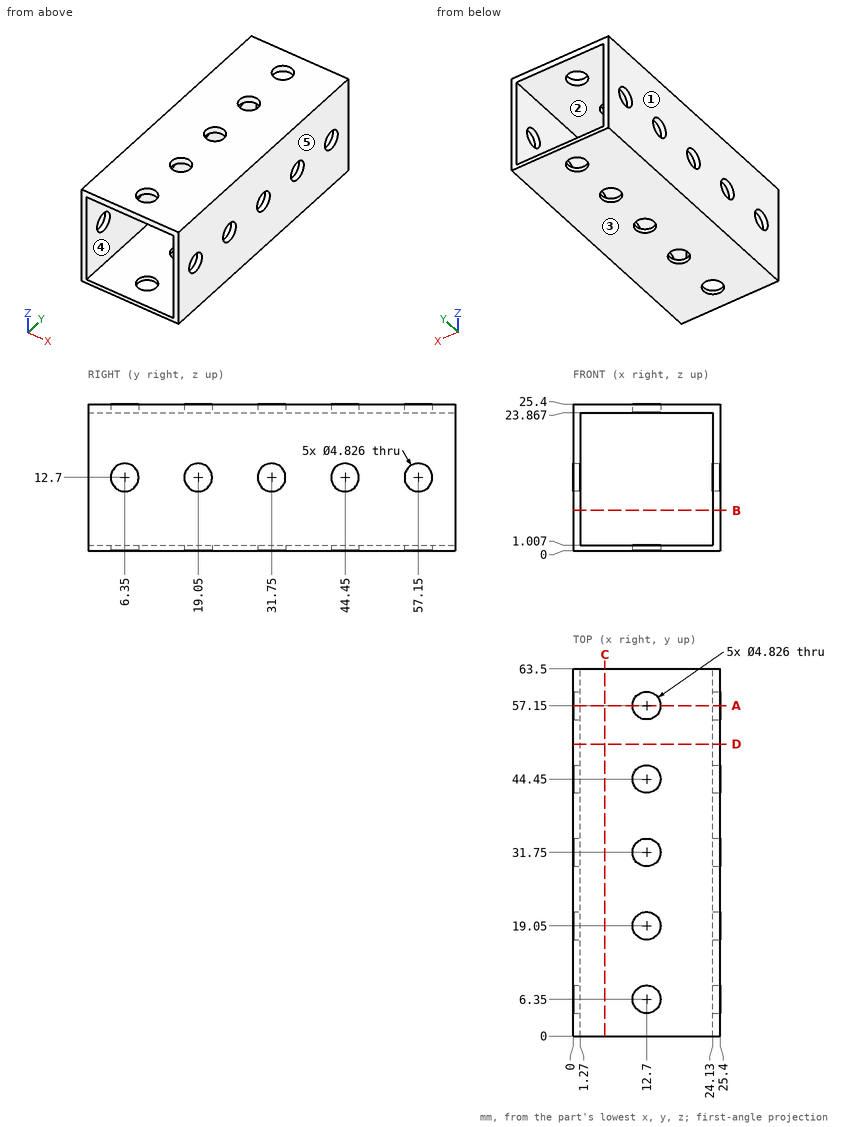
Could you check a few things on this drawing? It's one solid part, dimensions in mm from its lowest x, y, z. A direction names the side the tool comes from. Give positions to 0.01 mm unless a question says otherwise; leave off trailing zeros. Order: outer loops, then holes, each group sorted by start corner. A loop starts at its lowest first (then second) coordinate and runs counter-clockwise, first axis right, second up. Notation, with made-up numbers: (13.25, 39) -> (31.25, 39) arc R4 cw to (31.25, 43) -> close; hole circle Ø1 at (-17.75, 28). An arc over 180 degrees is marked (long way). Answer in a Markdown table with one row per item. Add a question column.
Item 1: Imagine slicing it at A-A (y = 57.15). List the corners of the cut face in (x, z) for me.
Item 2: For the marked faces 1 and 2, which set-ups out of +Z, -Z, +X, -X, +Y, -Y let a thin tool reach every point of the face, with its end or its side?
Item 3: I'm going to push a flat-ended pin straight in: P1, Ø4, axis at y = 31.75, z = 12.7, coming from the +X side. Where does the tip first touch, or does it pass through?
Item 4: Imagine slicing it at B-B (z = 7). List the corners of the cut face in (x, y) for me.
Item 5: We'd pull the mould along X, two halves only. Please class the marked faces 3, 4 and 5: pulls with the +X half, pulls with the -X half, needs draft (parallel to the pull), parting line crosses it, or undercut.
Item 6: Imagine slicing it at D-D (y = 50.5). List the corners of the cut face in (x, z) for me.
Item 7: Please list where these lines run through material, in increasing order: probe 1 along Z at (x, y) = (3.75, 37.5); probe 2 along X at (y, z) = (13.5, 16.75).
Item 8: Imagine slicing it at C-C (x = 5.5). List the corners of the cut face in (y, z) for me.
Result:
| question | item | result |
|---|---|---|
| 1 | outline | (0, 0) -> (10.29, 0) -> (10.29, 1.01) -> (1.27, 1.01) -> (1.27, 10.29) -> (0, 10.29) -> close; (0, 15.11) -> (1.27, 15.11) -> (1.27, 23.87) -> (10.29, 23.87) -> (10.29, 25.4) -> (0, 25.4) -> close; (15.11, 0) -> (25.4, 0) -> (25.4, 10.29) -> (24.13, 10.29) -> (24.13, 1.01) -> (15.11, 1.01) -> close; (15.11, 23.87) -> (24.13, 23.87) -> (24.13, 15.11) -> (25.4, 15.11) -> (25.4, 25.4) -> (15.11, 25.4) -> close |
| 2 | face 1 | +Z, -Z, -X, +Y, -Y |
| 2 | face 2 | +Y, -Y |
| 3 | P1 | through |
| 4 | outline | (0, 0) -> (1.27, 0) -> (1.27, 63.5) -> (0, 63.5) -> close; (24.13, 0) -> (25.4, 0) -> (25.4, 63.5) -> (24.13, 63.5) -> close |
| 5 | face 3 | needs draft |
| 5 | face 4 | undercut |
| 5 | face 5 | pulls with the +X half |
| 6 | outline | (0, 0) -> (25.4, 0) -> (25.4, 25.4) -> (0, 25.4) -> close; hole (1.27, 1.01) -> (24.13, 1.01) -> (24.13, 23.87) -> (1.27, 23.87) -> close |
| 7 | probe 1 | 0 to 1.01, 23.87 to 25.4 |
| 7 | probe 2 | 0 to 1.27, 24.13 to 25.4 |
| 8 | outline | (0, 0) -> (63.5, 0) -> (63.5, 1.01) -> (0, 1.01) -> close; (0, 23.87) -> (63.5, 23.87) -> (63.5, 25.4) -> (0, 25.4) -> close |
